```python
from build123d import *

# Parameters (mm, degrees)
BOSS_EXTRUDE1_DEPTH                              = 20
CUT_EXTRUDE1_DEPTH                               = 3
CUT_EXTRUDE3_DEPTH                               = 17
F_4_0MM_DOWEL_HOLE1_D                            = 4
F_4_0MM_DOWEL_HOLE1_DEPTH                        = 10
F_4_0MM_DOWEL_HOLE1_TIP                          = 1.201721238
M6X1_0_TAPPED_HOLE1_D                            = 5
CBORE_FOR_M5_HEX_HEAD_MACHINE_SCREW1_D           = 6.6
CBORE_FOR_M5_HEX_HEAD_MACHINE_SCREW1_CBORE_D     = 11
CBORE_FOR_M5_HEX_HEAD_MACHINE_SCREW1_CBORE_DEPTH = 10
F_4_0MM_DOWEL_HOLE2_D                            = 4


with BuildPart() as part:
    # Sketch1 → Boss-Extrude1 (new body)
    with BuildSketch(Plane(origin=(0, 0, 0), x_dir=(1, 0, 0), z_dir=(0, 1, 0))):
        Polygon((39, 30), (40, 29), (40, -29), (39, -30), (-39, -30), (-40, -29), (-40, 29), (-39, 30), align=None)
    extrude(amount=BOSS_EXTRUDE1_DEPTH)

    # Sketch2 → Cut-Extrude1 (cut)
    with BuildSketch(Plane(origin=(0, 20, 0), x_dir=(1, 0, 0), z_dir=(0, 1, 0))):
        with BuildLine():
            Line((-12.5, 7), (12.5, 7))
            ThreePointArc((12.5, 7), (19.5, 0), (12.5, -7))
            Line((12.5, -7), (-12.5, -7))
            ThreePointArc((-12.5, -7), (-19.5, 0), (-12.5, 7))
        make_face()
    extrude(amount=-CUT_EXTRUDE1_DEPTH, mode=Mode.SUBTRACT)

    # Sketch3 → Cut-Extrude3 (cut)
    with BuildSketch(Plane(origin=(0, 0, 0), x_dir=(-1, 0, 0), z_dir=(0, -1, 0))):
        with BuildLine():
            Line((13, -7.5), (-13, -7.5))
            ThreePointArc((-13, -7.5), (-20.5, 0), (-13, 7.5))
            Line((-13, 7.5), (13, 7.5))
            ThreePointArc((13, 7.5), (20.5, 0), (13, -7.5))
        make_face()
    extrude(amount=-CUT_EXTRUDE3_DEPTH, mode=Mode.SUBTRACT)

    # Ø4.0mm Dowel Hole1
    with Locations(Plane(origin=(0, 20, 0), x_dir=(1, 0, 0), z_dir=(0, 1, 0))):
        with Locations((9, 14), (-9, 14)):
            Hole(F_4_0MM_DOWEL_HOLE1_D / 2, depth=F_4_0MM_DOWEL_HOLE1_DEPTH)
            with Locations((0, 0, -(F_4_0MM_DOWEL_HOLE1_DEPTH + F_4_0MM_DOWEL_HOLE1_TIP / 2))):  # 118° drill point
                Cone(0, F_4_0MM_DOWEL_HOLE1_D / 2, F_4_0MM_DOWEL_HOLE1_TIP, mode=Mode.SUBTRACT)

    # M6x1.0 Tapped Hole1 (through all)
    with Locations(Plane(origin=(0, 20, 0), x_dir=(1, 0, 0), z_dir=(0, 1, 0))):
        with Locations((-32.5, 0), (32.5, 0)):
            Hole(M6X1_0_TAPPED_HOLE1_D / 2)

    # CBORE for M5 Hex Head Machine Screw1 (through all)
    with Locations(Plane(origin=(0, 20, 0), x_dir=(1, 0, 0), z_dir=(0, 1, 0))):
        with Locations((-32.5, -22.5), (-32.5, 22.5), (32.5, 22.5), (32.5, -22.5)):
            CounterBoreHole(CBORE_FOR_M5_HEX_HEAD_MACHINE_SCREW1_D / 2, CBORE_FOR_M5_HEX_HEAD_MACHINE_SCREW1_CBORE_D / 2, CBORE_FOR_M5_HEX_HEAD_MACHINE_SCREW1_CBORE_DEPTH)

    # Ø4.0mm Dowel Hole2 (through all)
    with Locations(Plane(origin=(0, 20, 0), x_dir=(1, 0, 0), z_dir=(0, 1, 0))):
        with Locations((32.5, 12.5), (32.5, -10), (-32.5, -10), (-32.5, 12.5)):
            Hole(F_4_0MM_DOWEL_HOLE2_D / 2)


solid = part.part
```
Input: part model. Units: mm. Frame: model coordinates. A direction names the side the tool comes from. Round coordinates to 2 decimals unless told otherwise and drop trailing zeros. Order: outer loops, then holes, each group sorted by start corner. A loop starts at its lowest first (then second) coordinate and runs counter-clockwise, first axis right, second up. Notation, with made-up numbers: (33, -38) - (41, -38) arc R14 cw to (41, -27) - close; hole circle Ø10 at (0.5, 40.25). An arc over 180 degrees is marked (long way). One line per question, with ' | ' between items. Start each with the question number.
1) Cut plane D-D, the plane x = -31.5. Give the number of separate pieces and of enclosed holes in the cut face, then the cut area to 3 significant figures.
2) Ray query, probe 1 along Z at (x, y) = (-32.5, 6.5); probe 2 along X at (y, z) = (4.75, -22.5); probe 3 along X at (y, z) = (9.5, -12.5). Return the intervals inside material, ascending.
3) Cut plane C-C, the plane z = -6. Return the cut outline in (x, y).
4) Cut plane B-B, the plane x = -5.5. Return the cut outline in (y, z).
5) Pull-direction query (Z, two-part tool) for faces 1 (the flat face through (1, 20, -14)), 2 (the cylindrical face through (9, 15, -16)), 3 (the flat face through (-1, 10, -30)); classes: +Z half, -Z half, draft (parallel to the pull), parting line (faces both ways), or undercut.
6) Set-up query: faces 4 (the cylindrical face through (20.5, 8.38, 0.16)), 5 (the flat face through (0, 19, -7)), 6 (the flat face through (1, 10, 30)), 7 (the cylindrical face through (-7.526, 14.93, -15.352)). Return all of +Z, -Z, +X, -X, +Y, -Y with unobstructed straight access to the full face (end or side cutting, diameter ignored); none if empty.
7) Cut plane A-A, the plane z = 22.5. Return the cut outline in (x, y).
8) Contact query for a flat-ended pin moving along its axis: P1, Ø10.5, axis at x = 32.5, z = -22.5, coming from the +Y side. Output: stop coordinate, or through.
Worked out:
1) separate pieces: 6 | enclosed holes: 0 | area: 628 mm^2
2) probe 1: z = -30 to -25.8, -19.2 to -14.5, -10.5 to -2.5, 2.5 to 8, 12 to 19.2, 25.8 to 30 | probe 2: x = -40 to -35.8, -29.2 to 29.2, 35.8 to 40 | probe 3: x = -40 to -34.5, -30.5 to 30.5, 34.5 to 40
3) outline: (-40, 0) - (-17.5, 0) - (-17.5, 17) - (-16.11, 17) - (-16.11, 20) - (-40, 20) - close; (16.11, 17) - (17.5, 17) - (17.5, 0) - (40, 0) - (40, 20) - (16.11, 20) - close
4) outline: (0, -30) - (20, -30) - (20, -7) - (17, -7) - (17, -7.5) - (0, -7.5) - close; (0, 7.5) - (17, 7.5) - (17, 7) - (20, 7) - (20, 30) - (0, 30) - close
5) face 1: draft | face 2: undercut | face 3: -Z half
6) face 4: -Y | face 5: +Y, -Y | face 6: +Z, +X, -X, +Y, -Y | face 7: +Y
7) outline: (-40, 0) - (-35.8, 0) - (-35.8, 10) - (-38, 10) - (-38, 20) - (-40, 20) - close; (-29.2, 0) - (29.2, 0) - (29.2, 10) - (27, 10) - (27, 20) - (-27, 20) - (-27, 10) - (-29.2, 10) - close; (35.8, 0) - (40, 0) - (40, 20) - (38, 20) - (38, 10) - (35.8, 10) - close
8) P1: stops at y = 10
